Here's how the part is built. I have some questions about the finished solid (model axes, mm). Face numbers are marked on the shaded views. Give positions to 0.01 mm unless a question says otherwise; leave off trailing zeros. Order: outer loops, then holes, each group sorted by start corner. A loop starts at its lowest first (then second) coordinate and runs counter-clockwise, first axis right, second up. Notation, with made-up numbers: (30.25, 33.25) -> (49.25, 33.25) arc R18 ccw to (49.25, 37.25) -> close; hole circle Ø1 at (50.5, 6.5). An arc over 180 degrees is marked (long way). Write each question's results on one line, items separated by ' | '. Start each with the question number.
Q1. Thinking about a two-plate mould opening in X: for the marked faces 1 and 2, which applies, pulls with the +X half, pulls with the -X half, needs draft (parallel to the pull), parting line crosses it, or undercut?
Q2. Imagine slicing it at A-A, the plane x = 0. Please give me the cut outline in (y, z).
Q3. I need wall thicknesses on line 1 along X through (y, z) = (-55, 66.5); line 2 along Z through (x, y) = (7.5, -49); line 3 along Z through (x, y) = (-35, -81.5). Which ranges of each line are inside material? Lowest first, please. Write a range as [from, to].
Q4. Imagine slicing it at D-D, the plane x = -34. Please give me the cut outline in (y, z), then the cut area to 3 significant figures.
Q5. Imagine slicing it at C-C, the plane y = -51.5. Please give me the cut outline in (x, z).
Q6. Imagine slicing it at B-B, the plane z = 38. Please give me the cut outline in (x, y).
Q7. I'm going to push flat-ended pins straight in: pin 1 (2 mm diameter, centred on x = 14, z = 52.5, fed in from +Y); pin 2 (5 mm diameter, centred on x = -5, y = -51.5, fed in from -Z); pin 3 (5 mm diameter, centred on x = -15.5, y = -79, fed in from -Z); pin 4 (12 mm diameter, centred on x = -23.5, y = -71.5, fed in from -Z). Where does each tip first touch, or does it pass through?
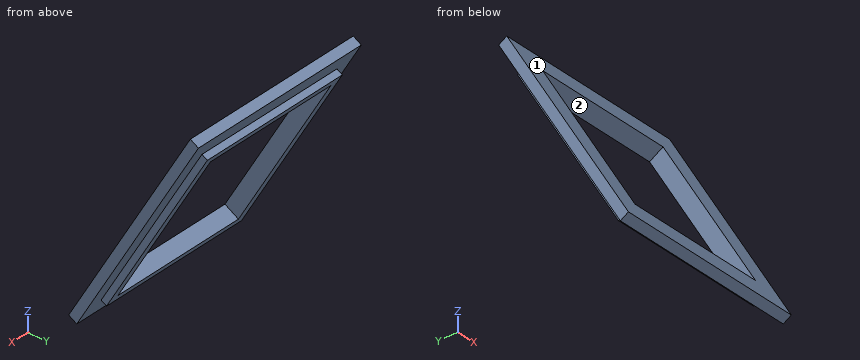
```python
from build123d import *

# Parameters (mm, degrees)
SKETCH1_W           = 60.6
SKETCH1_H           = 78.05786816
SKETCH1_W_2         = 44.8
SKETCH1_H_2         = 59.3
BOSS_EXTRUDE1_DEPTH = 3
SKETCH2_W           = 50.200000001
SKETCH2_H           = 64.7
SKETCH2_W_2         = 44.8
SKETCH2_H_2         = 59.299999999
BOSS_EXTRUDE2_DEPTH = 2


with BuildPart() as part:
    # Sketch1 → Boss-Extrude1 (new body)
    with BuildSketch(Plane(origin=(-8e-09, -784.034696128, -1198.711383076), x_dir=(1, 0, 0), z_dir=(0, 0.8660254037844385, -0.5000000000000002))):
        with Locations((-7.807791054, -1437.18747743)):
            Rectangle(SKETCH1_W, SKETCH1_H)
        with Locations((-7.807791055, -1437.183756537)):
            Rectangle(SKETCH1_W_2, SKETCH1_H_2, mode=Mode.SUBTRACT)
    extrude(amount=-BOSS_EXTRUDE1_DEPTH)

    # Sketch2 → Boss-Extrude2 (add)
    with BuildSketch(Plane(origin=(0, -68.968767322, 39.819136379), x_dir=(1, 0, 0), z_dir=(0, 0.8660254037844385, -0.5000000000000002))):
        with Locations((-7.807791061, -7.051898924)):
            Rectangle(SKETCH2_W, SKETCH2_H)
        with Locations((-7.807791063, -7.051898923)):
            Rectangle(SKETCH2_W_2, SKETCH2_H_2, mode=Mode.SUBTRACT)
    extrude(amount=BOSS_EXTRUDE2_DEPTH)


solid = part.part
```
Geometry check:
1) face 1: needs draft | face 2: undercut
2) outline: (-87.55, 13.63) -> (-84.96, 12.13) -> (-81.62, 17.91) -> (-79.89, 16.91) -> (-78.54, 19.25) -> (-82.87, 21.75) -> close; (-53.22, 73.1) -> (-48.89, 70.6) -> (-47.54, 72.94) -> (-49.27, 73.94) -> (-45.93, 79.73) -> (-48.52, 81.23) -> close
3) line 1: [-38.11, -30.21], [14.59, 22.49] | line 2: [70.67, 73.79], [74.41, 80.41] | line 3: [18.11, 24.11]
4) outline: (-87.55, 13.63) -> (-84.96, 12.13) -> (-45.93, 79.73) -> (-48.52, 81.23) -> close | area: 234 mm²
5) outline: (-38.11, 70.08) -> (-32.91, 70.08) -> (-32.91, 66.08) -> (-30.21, 66.08) -> (-30.21, 72.11) -> (14.59, 72.11) -> (14.59, 66.08) -> (17.29, 66.08) -> (17.29, 70.08) -> (22.49, 70.08) -> (22.49, 76.08) -> (-38.11, 76.08) -> close
6) outline: (-38.11, -73.48) -> (-30.21, -73.48) -> (-30.21, -67.71) -> (-32.91, -67.71) -> (-32.91, -70.02) -> (-38.11, -70.02) -> close; (14.59, -73.48) -> (22.49, -73.48) -> (22.49, -70.02) -> (17.29, -70.02) -> (17.29, -67.71) -> (14.59, -67.71) -> close
7) pin 1: y = -58.87 | pin 2: z = 70.67 | pin 3: z = 16.91 | pin 4: through
